from build123d import *

# Parameters (mm, degrees)
EXTRUDE_640_DEPTH      = 6.25
SKETCH_5_W             = 2.5
SKETCH_5_H             = 8
CUT_EXTRUDE_957_DEPTH  = 4.5
SKETCH_1_W             = 32.5
SKETCH_1_H             = 32.5
EXTRUDE_1522_DEPTH     = 3
SKETCH_4_R             = 1.5
CUT_EXTRUDE_1878_DEPTH = 34.669348078
SKETCH_9_R             = 2.5
CUT_EXTRUDE_4358_DEPTH = 2.5
FILLET_3_R             = 2.5
SKETCH_10_W            = 12.5
SKETCH_10_H            = 12.5
CUT_EXTRUDE_4764_DEPTH = 39.52353177
CUT_EXTRUDE_5191_REACH = 39.495
SKETCH_13_W            = 12.5
SKETCH_13_H            = 16
SKETCH_13_H_2          = 3.5
CHAMFER_3_SIZE         = 5
CHAMFER_3_SIZE_2       = 12.5
SKETCH_5338_R          = 1.1
CUT_EXTRUDE_5550_DEPTH = 8
CHAMFER_START          = -14
CHAMFER_4_DEPTH        = 4.5
EXTRUDE_6314_DEPTH     = 3.5
SKETCH_15_R            = 1
CUT_EXTRUDE_6618_DEPTH = 6
SKETCH_17_R            = 3.25
CUT_EXTRUDE_7180_DEPTH = 2.5


with BuildPart() as part:
    # Эскиз2 → Extrude 640 (new, symmetric)
    with BuildSketch(Plane.XY):
        Polygon((9.5, 16.25), (-14, 16.25), (-14, -16.25), (9.5, -16.25), (9.5, -11.75), (-9.5, -11.75), (-9.5, 11.75), (9.5, 11.75), align=None)
    extrude(amount=EXTRUDE_640_DEPTH, both=True)

    # Эскиз5 → Cut-Extrude 957 (cut)
    with BuildSketch(Plane.XZ.offset(11.75)):
        with Locations((-4.2, 2.25)):
            Rectangle(SKETCH_5_W, SKETCH_5_H)
    extrude(amount=CUT_EXTRUDE_957_DEPTH, mode=Mode.SUBTRACT)

    # Эскиз1 → Extrude 1522 (add)
    with BuildSketch(Plane(origin=(0, 0, -6.25), x_dir=(-1, 0, 0), z_dir=(0, 0, -1))):
        with Locations((-2.25, 0)):
            Rectangle(SKETCH_1_W, SKETCH_1_H)
    extrude(amount=EXTRUDE_1522_DEPTH)

    # Эскиз4 → Cut-Extrude 1878 (cut, through all)
    with BuildSketch(Plane(origin=(-9.5, 0, 0), x_dir=(0, 0, -1), z_dir=(1, 0, 0))):
        with Locations(Location((0, -5.77, 0), (0, 0, 90))):
            Circle(SKETCH_4_R)
    extrude(amount=-CUT_EXTRUDE_1878_DEPTH, mode=Mode.SUBTRACT)

    # Эскиз9 → Cut-Extrude 4358 (cut)
    with BuildSketch(Plane(origin=(0, 0, -9.25), x_dir=(-1, 0, 0), z_dir=(0, 0, -1))):
        with Locations((-11.75, 0)):
            Circle(SKETCH_9_R)
        with Locations((7.25, 0)):
            Circle(SKETCH_9_R)
    extrude(amount=-CUT_EXTRUDE_4358_DEPTH, mode=Mode.SUBTRACT)

    # Скругление3
    fillet_3_edges = [part.edges().sort_by_distance(p)[0] for p in [
        (14.25, 0, -6.75),
        (-4.75, 0, -6.75),
    ]]
    fillet(fillet_3_edges, radius=FILLET_3_R - 0.0001)  # a hair under: the kernel refuses the full size

    # Эскиз10 → Cut-Extrude 4764 (cut, through all)
    with BuildSketch(Plane(origin=(0, 16.25, 0), x_dir=(1, 0, 0), z_dir=(0, 1, 0))):
        with Locations((-3.25, 0)):
            Rectangle(SKETCH_10_W, SKETCH_10_H)
    extrude(amount=-CUT_EXTRUDE_4764_DEPTH, mode=Mode.SUBTRACT)

    # Эскиз13 → Cut-Extrude 5191 (cut, up to next)
    with BuildSketch(Plane.ZY.offset(14), mode=Mode.PRIVATE) as cut_extrude_5191_sk1:
        with Locations((0, 8.25)):
            Rectangle(SKETCH_13_W, SKETCH_13_H)
    cut_extrude_5191_tool1 = extrude(cut_extrude_5191_sk1.sketch, amount=-CUT_EXTRUDE_5191_REACH, mode=Mode.PRIVATE) & part.part
    # Эскиз13 → Cut-Extrude 5191 (cut, up to next)
    with BuildSketch(Plane.ZY.offset(14), mode=Mode.PRIVATE) as cut_extrude_5191_sk2:
        with Locations((0, -14.5)):
            Rectangle(SKETCH_13_W, SKETCH_13_H_2)
    cut_extrude_5191_tool2 = extrude(cut_extrude_5191_sk2.sketch, amount=-CUT_EXTRUDE_5191_REACH, mode=Mode.PRIVATE) & part.part
    add(cut_extrude_5191_tool1.solids().sort_by_distance((-14, 8.25, 0))[0], mode=Mode.SUBTRACT)
    add(cut_extrude_5191_tool2.solids().sort_by_distance((-14, -14.5, 0))[0], mode=Mode.SUBTRACT)

    # Фаска3
    # the kernel refuses this chamfer: 12.5, 5 mm, written as the material it adds along each edge
    with BuildSketch(Plane(origin=(3, 16.25, -6.25), x_dir=(-1, 0, 0), z_dir=(0, -1, 0))) as chamfer_3_piece_1:
        Polygon((CHAMFER_3_SIZE, 0), (0, -CHAMFER_3_SIZE_2), (0, 0), align=None)
    extrude(amount=4.5)
    with BuildSketch(Plane(origin=(3, 48.663920489, -6.25), x_dir=(-1, 0, 0), z_dir=(0, -1, 0))) as chamfer_3_piece_2_section:
        Polygon((CHAMFER_3_SIZE, 0), (0, -CHAMFER_3_SIZE_2), (0, 0), align=None)
    chamfer_3_piece_2 = extrude(amount=69.327840978, mode=Mode.PRIVATE)
    chamfer_3_piece_2 = split(chamfer_3_piece_2, bisect_by=Plane(origin=(3, -16.25, -6.25), z_dir=(0, 1, 0)), keep=Keep.TOP, mode=Mode.PRIVATE)
    chamfer_3_piece_2 = split(chamfer_3_piece_2, bisect_by=Plane(origin=(3, -11.75, -6.25), z_dir=(0, -1, 0)), keep=Keep.TOP, mode=Mode.PRIVATE)
    add(chamfer_3_piece_2)
    with BuildSketch(Plane(origin=(3, 20.663920489, -6.25), x_dir=(0, 0, 1), z_dir=(0, -1, 0))) as chamfer_3_piece_3_section:
        Polygon((CHAMFER_3_SIZE_2, 0), (0, CHAMFER_3_SIZE), (0, 0), align=None)
    chamfer_3_piece_3 = extrude(amount=69.327840978, mode=Mode.PRIVATE)
    chamfer_3_piece_3 = split(chamfer_3_piece_3, bisect_by=Plane(origin=(3, 11.75, -6.25), z_dir=(0, 1, 0)), keep=Keep.TOP, mode=Mode.PRIVATE)
    chamfer_3_piece_3 = split(chamfer_3_piece_3, bisect_by=Plane(origin=(3, 16.25, -6.25), z_dir=(0, -1, 0)), keep=Keep.TOP, mode=Mode.PRIVATE)
    add(chamfer_3_piece_3)
    with BuildSketch(Plane(origin=(3, -11.75, -6.25), x_dir=(0, 0, 1), z_dir=(0, -1, 0))) as chamfer_3_piece_4:
        Polygon((CHAMFER_3_SIZE_2, 0), (0, CHAMFER_3_SIZE), (0, 0), align=None)
    extrude(amount=4.5)
    with BuildSketch(Plane(origin=(-14, -12.75, -6.25), x_dir=(0, -1, 0), z_dir=(1, 0, 0))) as chamfer_3_piece_5_section:
        Polygon((CHAMFER_3_SIZE, 0), (0, -CHAMFER_3_SIZE_2), (0, 0), align=None)
    chamfer_3_piece_5 = extrude(amount=4.5, mode=Mode.PRIVATE)
    chamfer_3_piece_5 = split(chamfer_3_piece_5, bisect_by=Plane(origin=(-14, -16.25, -6.25), z_dir=(0, 1, 0)), keep=Keep.TOP, mode=Mode.PRIVATE)
    add(chamfer_3_piece_5)

    # Sketch 5338 → Cut-Extrude 5550 (cut)
    with BuildSketch(Plane(origin=(9.5, 0, 0), x_dir=(0, 0, -1), z_dir=(1, 0, 0))):
        with Locations((0, 13.7)):
            Circle(SKETCH_5338_R)
        with Locations((0, -13.7)):
            Circle(SKETCH_5338_R)
    extrude(amount=-CUT_EXTRUDE_5550_DEPTH, mode=Mode.SUBTRACT)

    # Фаска4: read off the stored shape, not the designer's step
    # Фаска4 outline → Фаска4 (add)
    with BuildSketch(Plane.YZ.offset(CHAMFER_START)):
        Polygon((0.25, -6.25), (4.75, -6.25), (0.25, 6.25), align=None)
    extrude(amount=CHAMFER_4_DEPTH)

    # Эскиз16 → Extrude 6314 (add)
    with BuildSketch(Plane.XY.offset(-6.25)):
        with BuildLine():
            Line((-14, 12.013932023), (-14, 16.25))
            Line((-14, 16.25), (-9.763932023, 16.25))
            ThreePointArc((-9.763932023, 16.25), (-9.878679656, 12.128679656), (-14, 12.013932023))
        make_face()
        with BuildLine():
            Line((14.263932023, 16.25), (18.5, 16.25))
            Line((18.5, 16.25), (18.5, 12.013932023))
            ThreePointArc((18.5, 12.013932023), (14.378679656, 12.128679656), (14.263932023, 16.25))
        make_face()
        with BuildLine():
            Line((18.5, -12.013932023), (18.5, -16.25))
            Line((18.5, -16.25), (14.263932023, -16.25))
            ThreePointArc((14.263932023, -16.25), (14.378679656, -12.128679656), (18.5, -12.013932023))
        make_face()
    extrude(amount=EXTRUDE_6314_DEPTH)

    # Эскиз15 → Cut-Extrude 6618 (cut)
    with BuildSketch(Plane(origin=(0, 0, -9.25), x_dir=(-1, 0, 0), z_dir=(0, 0, -1))):
        with Locations((12, -14.25)):
            Circle(SKETCH_15_R)
        with Locations((12, 14.25)):
            Circle(SKETCH_15_R)
        with Locations((-16.5, 14.25)):
            Circle(SKETCH_15_R)
        with Locations((-16.5, -14.25)):
            Circle(SKETCH_15_R)
    extrude(amount=-CUT_EXTRUDE_6618_DEPTH, mode=Mode.SUBTRACT)

    # Скругление4: read off the stored shape, not the designer's step
    # Скругление4 outline → Скругление4 (revolve, cut)
    with BuildSketch(Plane(origin=(16.5, 14.25, 0), x_dir=(1, 0, 0), z_dir=(0, -1, 0))):
        with BuildLine():
            ThreePointArc((1, -2.75), (2.414213562, -3.335786438), (3, -4.75))
            Line((3, -4.75), (3, -2.75))
            Line((3, -2.75), (1, -2.75))
        make_face()
    revolve(axis=Axis((16.5, 14.25, 0), (0, 0, 1)), mode=Mode.SUBTRACT)

    # Fillet 4 2 outline → Fillet 4 2 (revolve, cut)
    with BuildSketch(Plane(origin=(-12, 14.25, 0), x_dir=(1, 0, 0), z_dir=(0, -1, 0))):
        with BuildLine():
            ThreePointArc((1, -2.75), (2.414213562, -3.335786438), (3, -4.75))
            Line((3, -4.75), (3, -2.75))
            Line((3, -2.75), (1, -2.75))
        make_face()
    revolve(axis=Axis((-12, 14.25, 0), (0, 0, 1)), mode=Mode.SUBTRACT)

    # Fillet 4 3 outline → Fillet 4 3 (revolve, cut)
    with BuildSketch(Plane(origin=(16.5, -14.25, 0), x_dir=(1, 0, 0), z_dir=(0, -1, 0))):
        with BuildLine():
            ThreePointArc((1, -2.75), (2.414213562, -3.335786438), (3, -4.75))
            Line((3, -4.75), (3, -2.75))
            Line((3, -2.75), (1, -2.75))
        make_face()
    revolve(axis=Axis((16.5, -14.25, 0), (0, 0, 1)), mode=Mode.SUBTRACT)

    # Эскиз17 → Cut-Extrude 7180 (cut)
    with BuildSketch(Plane(origin=(-9.5, 0, 0), x_dir=(0, 0, -1), z_dir=(1, 0, 0))):
        with Locations((0, -5.77)):
            Circle(SKETCH_17_R)
    extrude(amount=-CUT_EXTRUDE_7180_DEPTH, mode=Mode.SUBTRACT)


solid = part.part
For this review, take the finished solid that the model builds, in its own axes (mm). A direction names the side the tool comes from. Give positions to 0.01 mm unless a question says otherwise; leave off trailing zeros. Order: outer loops, then holes, each group sorted by start corner. A loop starts at its lowest first (then second) coordinate and runs counter-clockwise, first axis right, second up. Notation, with made-up numbers: M 28,66.25 L 86,66.25 A27 ccw 86,101.25 Z; hole C 81.25,-28 d9. An arc over 180 degrees is marked long. Answer in a Markdown table with one row per item. Add a question column.
(1) Consider section D-D on y = 4. State the section outline as (x, z) points.
(2) Consider section C-C on z = -0.5. State the section outline as (x, y) points.
(3) Consider section B-B on x = 0. State the section outline as (y, z) points, and give its area (4 significant figures).
(4) For pin 1 (2.5 mm diameter, centred on x = 16.5, y = -14.25, fed in from -Z); pin 2 (3 mm diameter, centred on y = -2.5, z = 1, fed in from +X); pin 3 (2.5 mm diameter, centred on y = -14, z = 0, fed in from +X); pin 4 (10 mm diameter, centred on x = 4, y = -4, fed in from +Z), all flat-tipped, find the tip position at first contact; note any pin that passes through.
(5) Consider section A-A on y = -5.77. State the section outline as (x, z) points.
(6) For faces 1 (the face through (17, -14, -3.25)), 2 (the face through (5.56, 14.79, 0.14)), 3 (the face through (17, 14, -2.75)), list the 3-axis set-ups (+Z, -Z, +X, -X, +Y, -Y) from which the entire face can be reached by the end or side of a thin tool; tool diameter is ignored.
(7) Wall thickness on probe 1 along Y at (x, z) = (16.5, -7.35); probe 2 along Y at (x, z) = (7.5, 0); probe 3 along Y at (x, z) = (16.5, -5): over which ranges is each line inside the solid? List them lowest first. Write a range as [from, to].
(8) Mouldability with a two-part tool opening along Z and no side actions: class faces 4 (the face through (1.5, 14, 0)), 5 (the face through (2, 0, -6.25)), 6 (the face through (9.5, 15, 0)) as +Z half, -Z half, draft (parallel to the pull), parting line (faces both ways), or undercut.
Evaluation:
| question | item | result |
|---|---|---|
| 1 | outline | M -14,-9.25 L 18.5,-9.25 L 18.5,-6.25 L -9.5,-6.25 L -9.5,-4.17 L -14,-4.17 Z |
| 2 | outline | M -14,-15.45 L -9.5,-15.45 L -9.5,-8.98 L -12,-8.98 L -12,-7.18 L -14,-7.18 Z; M -14,-4.36 L -12,-4.36 L -12,-2.56 L -9.5,-2.56 L -9.5,2.68 L -14,2.68 Z; M 0.3,-16.25 L 9.5,-16.25 L 9.5,-14.68 L 1.5,-14.68 L 1.5,-12.72 L 9.5,-12.72 L 9.5,-11.75 L 0.3,-11.75 Z; M 0.3,11.75 L 9.5,11.75 L 9.5,12.72 L 1.5,12.72 L 1.5,14.68 L 9.5,14.68 L 9.5,16.25 L 0.3,16.25 Z |
| 3 | outline | M -16.25,-9.25 L 16.25,-9.25 L 16.25,-1.25 L 11.75,-1.25 L 11.75,-6.25 L -11.75,-6.25 L -11.75,-1.25 L -16.25,-1.25 Z |
| 3 | area | 142.5 mm^2 |
| 4 | pin 1 | stops at z = -9.25 |
| 4 | pin 2 | stops at x = -9.5 |
| 4 | pin 3 | stops at x = 9.5 |
| 4 | pin 4 | stops at z = -6.25 |
| 5 | outline | M -14,-9.25 L 18.5,-9.25 L 18.5,-6.25 L -9.5,-6.25 L -9.5,-3.25 L -12,-3.25 L -12,-1.5 L -14,-1.5 Z; M -14,1.5 L -12,1.5 L -12,3.25 L -9.5,3.25 L -9.5,6.25 L -14,6.25 Z |
| 6 | face 1 | -Z |
| 6 | face 2 | +X |
| 6 | face 3 | +Z, +X, +Y, -Y |
| 7 | probe 1 | y = [-16.25, -15.25], [-13.25, 13.25], [15.25, 16.25] |
| 7 | probe 2 | y = [-16.25, -14.8], [-12.6, -11.75], [11.75, 12.6], [14.8, 16.25] |
| 7 | probe 3 | y = [-16.25, -15.25], [-13.25, -11.25], [11.25, 13.25], [15.25, 16.25] |
| 8 | face 4 | undercut |
| 8 | face 5 | +Z half |
| 8 | face 6 | draft |
